Check sheet for the modelled part. Datum: model origin and axes. Units: mm. A direction names the side the tool comes from. Coordinates: 2 decimals unless noted, no trailing zeros. Loops run counter-clockwise (first coordinate to the right, second up) from the corner with the lowest first, then second, coordinate; pieces in that order, holes last.
```python
from build123d import *

# Parameters (mm, degrees)
SKETCH_2_W          = 23.5
SKETCH_2_H          = 18
EXTRUDE_1_DEPTH     = 12.5
SHELL_7_T           = 2
SKETCH_4_W          = 2
SKETCH_4_H          = 3.5
CUT_EXTRUDE_3_DEPTH = 35.734708866
SKETCH_8_W          = 14.567673111
SKETCH_8_H          = 27.5
CUT_EXTRUDE_5_DEPTH = 2
SKETCH_7_R          = 3.5
EXTRUDE_2_DEPTH     = 5


with BuildPart() as part:
    # Эскиз2 → Бобышка-Вытянуть1 (new body)
    with BuildSketch(Plane(origin=(0, 0, 0), x_dir=(0, 0, -1), z_dir=(1, 0, 0))):
        with Locations((-11.75, 9)):
            Rectangle(SKETCH_2_W, SKETCH_2_H)
    extrude(amount=EXTRUDE_1_DEPTH)

    # Оболочка7
    shell_7_openings = [part.faces().sort_by_distance(p)[0] for p in [
        (12.5, 9, 11.75),
    ]]
    offset(amount=SHELL_7_T, openings=shell_7_openings, kind=Kind.INTERSECTION)

    # Эскиз4 → Вырез-Вытянуть3 (cut, through all)
    with BuildSketch(Plane(origin=(0, 0, 0), x_dir=(0, 0, -1), z_dir=(1, 0, 0))):
        with Locations((1, 5.25)):
            Rectangle(SKETCH_4_W, SKETCH_4_H)
    extrude(amount=CUT_EXTRUDE_3_DEPTH, mode=Mode.SUBTRACT)

    # Эскиз8 → Вырез-Вытянуть5 (cut)
    with BuildSketch(Plane(origin=(0, 20, 0), x_dir=(1, 0, 0), z_dir=(0, 1, 0))):
        with Locations((5.283836556, -11.75)):
            Rectangle(SKETCH_8_W, SKETCH_8_H)
    extrude(amount=-CUT_EXTRUDE_5_DEPTH, mode=Mode.SUBTRACT)

    # Эскиз7 → Бобышка-Вытянуть2 (add)
    with BuildSketch(Plane.XZ.offset(2)):
        with Locations(Location((5.25, 5, 0), (0, 0, 90))):
            Circle(SKETCH_7_R)
    extrude(amount=EXTRUDE_2_DEPTH)


solid = part.part
```
1) Set-up check for faces 1 (the cylindrical face through (6.591, -4.465, 8.233)), 2 (the flat face through (6, 3.5, -1)), 3 (the flat face through (6, 9, 23.5)), 4 (the flat face through (12.5, -1, 16)): record each of +Z, -Z, +X, -X, +Y, -Y from which the full face is reachable in a straight line by a thin tool's end or side.
Answer sheet:
face 1: -Y
face 2: -Z, +X
face 3: +X, +Y
face 4: +Z, -Z, +X, +Y, -Y
2) Section check C-C on z = 5. Enter the section's corners in (x, y), plus the area to 3 significant figures.
Answer sheet:
outline: (-2, -2) - (1.75, -2) - (1.75, -7) - (8.75, -7) - (8.75, -2) - (12.5, -2) - (12.5, 0) - (0, 0) - (0, 18) - (-2, 18) - close
area: 100 mm2
3) Section check A-A on x = 5.25. Enter the section's corners in (y, z).
Answer sheet:
outline: (-7, 1.5) - (-2, 1.5) - (-2, -2) - (3.5, -2) - (3.5, 0) - (0, 0) - (0, 23.5) - (18, 23.5) - (18, 25.5) - (-2, 25.5) - (-2, 8.5) - (-7, 8.5) - close; (7, -2) - (18, -2) - (18, 0) - (7, 0) - close
4) Section check D-D on x = 2.5. Enter the section's corners in (y, z), plus the area to 3 significant figures.
Answer sheet:
outline: (-7, 2.83) - (-2, 2.83) - (-2, -2) - (3.5, -2) - (3.5, 0) - (0, 0) - (0, 23.5) - (18, 23.5) - (18, 25.5) - (-2, 25.5) - (-2, 7.17) - (-7, 7.17) - close; (7, -2) - (18, -2) - (18, 0) - (7, 0) - close
area: 142 mm2
5) Depth check by flat-ended pin: pin 1 (7 mm diameter, centred on x = 4, z = 17.5, fed in from -Y); pin 2 (5.5 mm diameter, centred on y = 11, z = 7, fed in from +X); pin 3 (1 mm diameter, centred on x = 5.5, z = 6.5, fed in from +Y). Enter the tip coordinate at first touch or a pass-through.
Answer sheet:
pin 1: stops at y = -2
pin 2: stops at x = 0
pin 3: stops at y = 0
6) Section check B-B on y = 0.75. Enter the section's corners in (x, z).
Answer sheet:
outline: (-2, -2) - (12.5, -2) - (12.5, 0) - (0, 0) - (0, 23.5) - (12.5, 23.5) - (12.5, 25.5) - (-2, 25.5) - close
7) Scan lines: line 1 (Z direction, x = 7, y = 1.5); line 2 (Y direction, x = 10.5, z = -0.5); line 3 (X direction, y = 2.75, z = 16.5). Record each from-to range of solid material in increasing order.
Answer sheet:
line 1: z = -2 to 0, 23.5 to 25.5
line 2: y = -2 to 3.5, 7 to 18
line 3: x = -2 to 0
